from build123d import *

# Parameters (mm, degrees)
ESQUISSE1_W             = 203.2
ESQUISSE1_H             = 32
BOSS_EXTRU_1_DEPTH      = 6
ESQUISSE2_W             = 203.2
ESQUISSE2_H             = 36
BOSS_EXTRU_2_DEPTH      = 6
ESQUISSE3_R             = 7.5
ESQUISSE3_R_2           = 4.5
ESQUISSE3_R_3           = 1.75
ENL_V_MAT_EXTRU_1_DEPTH = 113.545812894
ESQUISSE6_W             = 203.2
ESQUISSE6_H             = 50
BOSS_EXTRU_4_DEPTH      = 6
BOSS_EXTRU_5_DEPTH      = 6
CONG_3_R                = 3
CONG_4_R                = 10
D_GAGEMENT_M31_D        = 3.2
D_GAGEMENT_M31_DEPTH    = 6
D_GAGEMENT_M31_TIP      = 0.96137699
ESQUISSE11_R            = 3.2385
ENL_V_MAT_EXTRU_3_DEPTH = 6
D_GAGEMENT_M32_D        = 3.2
D_GAGEMENT_M32_DEPTH    = 6
D_GAGEMENT_M32_TIP      = 0.96137699


with BuildPart() as part:
    # Esquisse1 → Boss.-Extru.1 (new body)
    with BuildSketch(Plane.XY):
        Rectangle(ESQUISSE1_W, ESQUISSE1_H)
    extrude(amount=BOSS_EXTRU_1_DEPTH)

    # Esquisse2 → Boss.-Extru.2 (add)
    with BuildSketch(Plane(origin=(0, 16, 0), x_dir=(1, 0, 0), z_dir=(0, 1, 0))):
        with Locations((0, 12)):
            Rectangle(ESQUISSE2_W, ESQUISSE2_H)
    extrude(amount=BOSS_EXTRU_2_DEPTH)

    # Esquisse3 → Enlèv. mat.-Extru.1 (cut, through all)
    with BuildSketch(Plane(origin=(0, 22, 0), x_dir=(1, 0, 0), z_dir=(0, 1, 0))):
        with Locations(Location((-73.6, 11, 0), (0, 0, 270))):
            Circle(ESQUISSE3_R)
        with Locations(Location((73.6, 11, 0), (0, 0, 270))):
            Circle(ESQUISSE3_R)
        with Locations(Location((0, 15, 0), (0, 0, 270))):
            Circle(ESQUISSE3_R_2)
        with Locations(Location((0, 23, 0), (0, 0, 270))):
            Circle(ESQUISSE3_R_3)
        with Locations(Location((0, 7, 0), (0, 0, 270))):
            Circle(ESQUISSE3_R_3)
        with Locations(Location((8, 15, 0), (0, 0, 270))):
            Circle(ESQUISSE3_R_3)
        with Locations(Location((-8, 15, 0), (0, 0, 270))):
            Circle(ESQUISSE3_R_3)
    extrude(amount=-ENL_V_MAT_EXTRU_1_DEPTH, mode=Mode.SUBTRACT)

    # Esquisse6 → Boss.-Extru.4 (add)
    with BuildSketch(Plane.XZ.offset(16)):
        with Locations((0, 25)):
            Rectangle(ESQUISSE6_W, ESQUISSE6_H)
    extrude(amount=BOSS_EXTRU_4_DEPTH)

    # Esquisse7 → Boss.-Extru.5 (add)
    with BuildSketch(Plane(origin=(101.6, 0, 0), x_dir=(0, 0, -1), z_dir=(1, 0, 0))):
        Polygon((-50, -16), (-6, 22), (0, 22), (0, -16), align=None)
    boss_extru_5 = extrude(amount=-BOSS_EXTRU_5_DEPTH)

    # Symétrie1: Boss.-Extru.5 across plane
    add(boss_extru_5.mirror(Plane(origin=(0, 0, 0), x_dir=(0, 0, 1), z_dir=(1, 0, 0))))

    # Congé3
    cong_3_edges = [part.edges().sort_by_distance(p)[0] for p in [
        (0, -16, 6),
        (0, -22, 0),
    ]]
    fillet(cong_3_edges, radius=CONG_3_R)

    # Congé4
    cong_4_edges = [part.edges().sort_by_distance(p)[0] for p in [
        (101.6, 19, -30),
        (-101.6, 19, -30),
    ]]
    fillet(cong_4_edges, radius=CONG_4_R)

    # Dégagement M31
    with Locations(Plane(origin=(85.6, 11.7, 0), x_dir=(-1, 0, 0), z_dir=(0, 0, -1))):
        with Locations((0, 0), (24, 0), (0, -21.4), (24, -21.4), (147.2, 0), (171.2, 0), (147.2, -21.4), (171.2, -21.4)):
            Hole(D_GAGEMENT_M31_D / 2, depth=D_GAGEMENT_M31_DEPTH)
            with Locations((0, 0, -(D_GAGEMENT_M31_DEPTH + D_GAGEMENT_M31_TIP / 2))):  # 118° drill point
                Cone(0, D_GAGEMENT_M31_D / 2, D_GAGEMENT_M31_TIP, mode=Mode.SUBTRACT)

    # Esquisse11 → Enlèv. mat.-Extru.3 (cut)
    with BuildSketch(Plane.XZ.offset(22)):
        with Locations(Location((38.1, 30.95, 0), (0, 0, 270))):
            Circle(ESQUISSE11_R)
    extrude(amount=-ENL_V_MAT_EXTRU_3_DEPTH, mode=Mode.SUBTRACT)

    # Dégagement M32
    with Locations(Plane(origin=(-70.62, -16, 17.48), x_dir=(0, 0, 1), z_dir=(0, 1, 0))):
        with Locations((0, 0), (26.94, 0), (0, 141.24), (26.94, 141.24)):
            Hole(D_GAGEMENT_M32_D / 2, depth=D_GAGEMENT_M32_DEPTH)
            with Locations((0, 0, -(D_GAGEMENT_M32_DEPTH + D_GAGEMENT_M32_TIP / 2))):  # 118° drill point
                Cone(0, D_GAGEMENT_M32_D / 2, D_GAGEMENT_M32_TIP, mode=Mode.SUBTRACT)


solid = part.part
Can you work these out from the model? Positions are in its coordinate system, mm. A direction names the side the tool comes from. Give positions to 0.01 mm unless a question says otherwise; leave off trailing zeros. Order: outer loops, then holes, each group sorted by start corner. A loop starts at its lowest first (then second) coordinate and runs counter-clockwise, first axis right, second up. Notation, with made-up numbers: M 6.25,10.5 L 42.25,10.5 A24 cw 42.25,25.5 Z; hole C -24,72 d3. An arc over 180 degrees is marked long. Use a Markdown table: item, result. Add a question column.
Item 1: If I drill on L1, parallel to X at y = -20.2, z = 17.48; L2, parallel to X at y = 11.7, z = 2.2; L3, parallel to Z at x = 70.62, y = -19.7, over which ranges is the centre line in solid material (lowest first)? Write a range as [from, to].
Item 2: Suppose I cut it at A-A (x = 21.5). List the corners of the cut face in (y, z) for me.
Item 3: We'd pull the mould along Z, two halves only. Please class faces 3 (the flat face through (-1, -16, 30)), 4 (the flat face through (-1, -1, 0)), 5 (the cylindrical face through (66.946, 19.042, -7.539)), 6 (the flat face through (-1, 4, 6)): +Z half, -Z half, draft (parallel to the pull), parting line (faces both ways), or undercut.
Item 4: Suppose I cut it at D-D (z = 41). List the corners of the cut face in (x, y) for me.
Item 5: Will these pins go through, and if not, where does the flat tip stop? pin 1 (12 mm diameter, centred on x = -74.5, y = 8.5, fed in from +Z); pin 2 (17 mm diameter, centred on x = -73.6, z = -11, fed in from +Y); pin 3 (10 mm diameter, centred on x = -36, y = 4, fed in from -Z); pin 4 (2 mm diameter, centred on x = 0, z = -7, fed in from -Y).
Item 6: Suppose I cut it at C-C (y = 2). List the corners of the cut face in (x, z) for me, then the cut area to 3 significant figures.
Item 7: For faces 1 (the flat face through (95.6, -5, 18)), 2 (the flat face through (-1, 19, -30)), which set-ups out of +Z, -Z, +X, -X, +Y, -Y let a thin tool reach every point of the face, with its end or its side?
Item 8: Suppose I cut it at B-B (z = 30). List the corners of the cut face in (x, y) for me.
Answer sheet:
| question | item | result |
|---|---|---|
| 1 | L1 | x = [-101.6, -72.22], [-69.02, 69.02], [72.22, 101.6] |
| 1 | L2 | x = [-101.6, -87.2], [-84, -63.2], [-60, 60], [63.2, 84], [87.2, 101.6] |
| 1 | L3 | z = [0.08, 15.88], [19.08, 42.82], [46.02, 50] |
| 2 | outline | M -22,3 A3 ccw -19,0 L 16,0 L 16,-30 L 22,-30 L 22,6 L -13,6 A3 cw -16,9 L -16,50 L -22,50 Z |
| 3 | face 3 | draft |
| 3 | face 4 | -Z half |
| 3 | face 5 | undercut |
| 3 | face 6 | +Z half |
| 4 | outline | M -101.6,-22 L 101.6,-22 L 101.6,-8.23 L 95.6,-8.23 L 95.6,-16 L -95.6,-16 L -95.6,-8.23 L -101.6,-8.23 Z |
| 5 | pin 1 | stops at z = 6 |
| 5 | pin 2 | stops at y = 22 |
| 5 | pin 3 | stops at z = 0 |
| 5 | pin 4 | passes through |
| 6 | outline | M -101.6,0 L 101.6,0 L 101.6,29.16 L 95.6,29.16 L 95.6,6 L -95.6,6 L -95.6,29.16 L -101.6,29.16 Z |
| 6 | area | 1,500 mm² |
| 7 | face 1 | +Z, +Y |
| 7 | face 2 | -Z, +X, -X, +Y, -Y |
| 8 | outline | M -101.6,-22 L 35,-22 L 35,-16 L -95.6,-16 L -95.6,1.27 L -101.6,1.27 Z; M 41.2,-22 L 101.6,-22 L 101.6,1.27 L 95.6,1.27 L 95.6,-16 L 41.2,-16 Z |
